```python
from build123d import *

# Parameters (mm, degrees)
F0_R     = 1.55
F1_DEPTH = 2
F2_W     = 12.2
F2_H     = 16.5
F3_DEPTH = 11
F2_W_2   = 10.6
F2_H_2   = 10
F4_DEPTH = 17
F5_SIZE  = 5
F2_W_3   = 9
F2_H_3   = 20.2
F6_DEPTH = 9


with BuildPart() as f1:
    # F0 (on Top) → F1 (new body)
    with BuildSketch(Plane.XY):
        with BuildLine():
            Line((50, 45), (-50, 45))
            ThreePointArc((-50, 45), (-53.535534, 43.535534), (-55, 40))
            Line((-55, 40), (-55, -40))
            ThreePointArc((-55, -40), (-53.535534, -43.535534), (-50, -45))
            Line((-50, -45), (50, -45))
            ThreePointArc((50, -45), (53.535534, -43.535534), (55, -40))
            Line((55, -40), (55, 40))
            ThreePointArc((55, 40), (53.535534, 43.535534), (50, 45))
        make_face()
        with Locations((-50, -40)):
            Circle(F0_R, mode=Mode.SUBTRACT)
        with Locations((50, -40)):
            Circle(F0_R, mode=Mode.SUBTRACT)
        with Locations((-50, 40)):
            Circle(F0_R, mode=Mode.SUBTRACT)
        with Locations((50, 40)):
            Circle(F0_R, mode=Mode.SUBTRACT)
    extrude(amount=F1_DEPTH)

    # F2 (on Top) → F3 (join)
    with BuildSketch(Plane.XY):
        with Locations((32.9, -40.95)):
            Rectangle(F2_W, F2_H)
    extrude(amount=-F3_DEPTH)

    # F2 (on Top) → F4 (join)
    with BuildSketch(Plane.XY):
        with Locations((44.7, -32)):
            Rectangle(F2_W_2, F2_H_2)
    extrude(amount=-F4_DEPTH)

    # F5
    f5_edges = [f1.edges().sort_by_distance(p)[0] for p in [
        (50, -32, -17),
    ]]
    chamfer(f5_edges, length=F5_SIZE)

    # F2 (on Top) → F6 (join)
    with BuildSketch(Plane.XY):
        with Locations((-48.1, -25.9)):
            Rectangle(F2_W_3, F2_H_3)
        with Locations((-48.1, -4.9)):
            Rectangle(F2_W_3, F2_H_3)
    extrude(amount=-F6_DEPTH)


solid = f1.part
```
Work out the finished part from the listing and answer in its coordinate system (mm). A direction names the side the tool comes from. Give positions to 0.01 mm unless a question says otherwise; leave off trailing zeros. Order: outer loops, then holes, each group sorted by start corner. A loop starts at its lowest first (then second) coordinate and runs counter-clockwise, first axis right, second up. Notation, with made-up numbers: (-2.75, 65.5) -> (21.25, 65.5) arc R13 ccw to (21.25, 79.5) -> close; hole circle Ø1 at (3.25, 54.5). An arc over 180 degrees is marked (long way). Answer as CSV lines item,"result". Start each with the question number.
(1) Section D-D, the plane z = -13.5 is taken. Write down the section's boundary in (x, y).
(2) Section A-A, the plane z = -7.75 is taken. Write down the section's boundary in (x, y), plus the area to 3 significant figures.
(3) Each of these flat-tipped pins is pushed along its axis until it touches: pin 1 Ø10 at (y, z) = (-15, -14.5) entering from +X; pin 2 Ø5 at (x, y) = (-2.5, 11) entering from -Z; pin 3 Ø8 at (y, z) = (-12.5, -10) entering from -X; pin 4 Ø13.5 at (x, y) = (36, -44) entering from -Z. Where does it stop, or does it pass through?
(4) For a pull along Y with two mould halves and no side action, classify faces 4 (the flat face through (-48, -36, -4)), 5 (the flat face through (-43.6, -26, -4)), 6 (the flat face through (-48, -15, -4)) as released by +Y, released by -Y, zero draft, split by the parting line, or undercut.
(5) Section B-B, the plane x = 32 is taken. Write down the section's boundary in (y, z).
(6) Section C-C, the plane y = 21 is taken. Write down the section's boundary in (x, z), plus the area to 3 significant figures.
(7) Which of the six approach directions +Z, -Z, +X, -X, +Y, -Y give full straight-line access (tool end or side, diameter ignored) to faces 1 (the flat face through (39, -41, -5)), 2 (the flat face through (-52.6, -5, -4)), 3 (the flat face through (-48, -15.8, -4))?
(8) Consider line 1 along Y through (x, z) = (-50, 0.75); line 2 along Z through (x, y) = (-43, 38.5); line 3 along X through (y, z) = (-12, -8). Determine where each line is inside the solid, lowest interval first.
Entries:
1,outline,"(39.4, -37) -> (48.5, -37) -> (48.5, -27) -> (39.4, -27) -> close"
2,outline,"(-52.6, -36) -> (-43.6, -36) -> (-43.6, -15.8) -> (-52.6, -15.8) -> close; (-52.6, -15) -> (-43.6, -15) -> (-43.6, 5.2) -> (-52.6, 5.2) -> close; (26.8, -49.2) -> (39, -49.2) -> (39, -32.7) -> (26.8, -32.7) -> close; (39.4, -37) -> (50, -37) -> (50, -27) -> (39.4, -27) -> close"
2,area,"671 mm²"
3,pin 1,"through"
3,pin 2,"z = 0"
3,pin 3,"x = -52.6"
3,pin 4,"z = -11"
4,face 4,"released by -Y"
4,face 5,"zero draft"
4,face 6,"undercut"
5,outline,"(-49.2, -11) -> (-32.7, -11) -> (-32.7, 0) -> (45, 0) -> (45, 2) -> (-45, 2) -> (-45, 0) -> (-49.2, 0) -> close"
6,outline,"(-55, 0) -> (55, 0) -> (55, 2) -> (-55, 2) -> close"
6,area,"220 mm²"
7,face 1,"-Z, +Y, -Y"
7,face 2,"-Z, -X, +Y, -Y"
7,face 3,"-Z, +X, -X"
8,line 1,"-45 to -41.55, -38.45 to 38.45, 41.55 to 45"
8,line 2,"0 to 2"
8,line 3,"-52.6 to -43.6"
